Autodesk Inventor part; units mm, degrees
ref_plane "Work Plane1" through (-8.617, 4.975, 0) normal (-0.5, -0.8660254, 0) x (0, 0, -1)
ref_plane "YZ Plane" through (0, 0, 0) normal (1, 0, 0) x (0, 1, 0)
ref_plane "XZ Plane" through (0, 0, 0) normal (0, 1, 0) x (-1, 0, 0)
sketch "Sketch1" plane through (0, 0, 0) normal (0, 0, 1) x (1, 0, 0)
  circle A0 centre (0, 0) radius 30
  circle A1 centre (0, 0) radius 40
  circle A2 centre (0, 0) radius 25
  circle A3 centre (0, 0) radius 13
  circle A4 centre (0, 0) radius 5.5
  circle A5 centre (0, 0) radius 9.95 construction
  line L0 (0, 9.95) -> (8.617, 4.975)
  line L1 (8.617, 4.975) -> (8.617, -4.975)
  line L2 (8.617, -4.975) -> (0, -9.95)
  line L3 (0, -9.95) -> (-8.617, -4.975)
  line L4 (-8.617, -4.975) -> (-8.617, 4.975)
  line L5 (-8.617, 4.975) -> (0, 9.95)
  line L6 (0, 9.95) -> (0, -9.95) construction
  dimension "bolt_head_hub_WAC" = 19.9
  dimension "wheel_diam" = 60
  dimension "d1" = 80
  dimension "d4" = 50
  dimension "d5" = 26
  dimension "hub_id" = 11
extrude "Extrusion1" add sketch "Sketch1" along normal blind 3 contours A0 | A1 | A2 | A3 | A4 | L0 L1 L2 L3 L4 L5
extrude "Extrusion2" add sketch "Sketch1" along normal blind 28 contours A0
extrude "Extrusion3" add sketch "Sketch1" along normal blind 18 contours A3 | L0 L1 L2 L3 L4 L5
extrude "Extrusion4" cut sketch "Sketch1" against normal blind 8.4 from surface at 18 contours L0 L1 L2 L3 L4 L5
extrude "Extrusion5" cut sketch "Sketch1" along normal up to surface (3 mm away) contours A4
fillet "Fillet1" radius 2 1 edges at (-30, 0, 3)
ref_plane "Work Plane1" through (-8.617, 4.975, 0) normal (-0.5, -0.8660254, 0) x (0, 0, -1)
sketch "Sketch3" plane through (-8.617, 4.975, 0) normal (-0.5, -0.8660254, 0) x (0, 0, -1)
  line L0 (-3, 22.95) -> (-18, 22.95)
  line L1 (-3, 34.95) -> (-3, -15.05)
  line L2 (-3, -3.05) -> (-3, 22.95)
  line L3 (-28, 34.95) -> (-3, 34.95)
  line L4 (-18, 22.95) -> (-3, 22.95)
  line L5 (-3, 22.95) -> (-3, 19.95)
  line L6 (-3, 19.95) -> (-18, 19.95)
  line L7 (-18, 19.95) -> (-18, 22.95)
  arc A0 (-18, 22.95) -> (-28, 34.95) centre (-32.838, 20.7516) ccw
  point P0 (0, 9.95)
  dimension "d18" = 3
  dimension "d21" = 15
extrude "Extrusion6" add sketch "Sketch3" along normal mid plane 3
pattern_circular "Circular Pattern1" count 4 over 360 about axis through (0, 0, -10) along (0, 0, 1) of "Extrusion6"
equation "\"bolt_head_hub_WAC\" = bolt_WAC + 2 * printer_tolerance"
equation "\"d1\" = wheel_diam + 2 * flange_extra"
equation "\"d4\" = wheel_diam - 2 * wheel_thick"
equation "\"d5\" = bolt_head_hub_WAC + 2 * bolt_head_hub_clearance"
equation "\"hub_id\" = bolt_od + 2 * printer_tolerance"
equation "\"d8\" = track_w + flange_w"
equation "\"d10\" = flange_w + hub_height"
equation "\"track_w\" = 25"
equation "\"wheel_thick\" = 5"
equation "\"bolt_head_hub_clearance\" = 3.05"
equation "\"hub_height\" = 15"
equation "\"bolt_head_thick\" = 6.4"
equation "\"bolt_WAC\" = 18.9"
equation "\"printer_tolerance\" = 0.5"
properties part number "test_wheel_v1"
CAD build for the part. Positions are in the model's coordinates, mm. Give positions to 0.01 mm unless a question says otherwise; leave off trailing zeros. Order: outer loops, then holes, each group sorted by start corner. A loop starts at its lowest first (then second) coordinate and runs counter-clockwise, first axis right, second up. Notation, with made-up numbers: M -37.75,-6 L -8.75,-6 A17 cw -8.75,22 Z; hole C 10.25,80.5 d3. An arc over 180 degrees is marked long. Put each result on its own line as item: value. Start each with the question number.
(1) Saw through at D-D, the plane z = 19. Write the cut outline in (x, y), then the cut area to 3 significant figures.
(2) Saw through at A-A, the plane z = 7. Write the cut outline in (x, y).
(3) Saw through at B-B, the plane y = 0. Write the cut outline in (x, z).
(4) Saw through at C-C, the plane z = 11.25. Write the cut outline in (x, y) (3 decimals).
(5) Drill centre lines: line 1 along Y through (x, z) = (0, 7.25); line 2 along Y through (x, z) = (-0.5, 21.25) (3 decimals); line 3 along X through (y, z) = (0.5, 10.25) (3 decimals). Where is each one in solid material? Low to high.
(6) Flat gauge pins, fed straight in: pin 1 Ø1 at (x, y) = (-24, 24) entering from +Z; pin 2 Ø10 at (y, z) = (-6.5, 3.5) entering from +X; pin 3 Ø3 at (x, z) = (7.5, 12.5) entering from +Y. Where does each tip first touch, or does it go through?
(7) Mould opens along Y. For faces 1 (the flat face through (-9, 0, 18)), 2 (the cylindrical face through (-8.67, 39.05, 1.48)) say: +Y half, -Y half, draft (parallel to the pull), parting line (faces both ways), or undercut.
Check result:
1. outline: C 0,0 d60; hole M -22.36,11.18 A25 ccw -13.78,-20.86 L -9.59,-13.62 L -7,-15.12 L -11.18,-22.36 A25 ccw 20.86,-13.78 L 13.62,-9.59 L 15.12,-7 L 22.36,-11.18 A25 ccw 13.78,20.86 L 9.59,13.62 L 7,15.12 L 11.18,22.36 A25 ccw -20.86,13.78 L -13.62,9.59 L -15.12,7 Z
1. area: 965 mm2
2. outline: C 0,0 d60; hole M -22.36,11.18 A25 ccw -13.78,-20.86 L -7.76,-10.43 A13 cw -11.93,5.16 Z; hole M -20.86,13.78 L -10.43,7.76 A13 cw 5.16,11.93 L 11.18,22.36 A25 ccw Z; hole M -11.18,-22.36 A25 ccw 20.86,-13.78 L 10.43,-7.76 A13 cw -5.16,-11.93 Z; hole C 0,0 d11; hole M 7.76,10.43 A13 cw 11.93,-5.16 L 22.36,-11.18 A25 ccw 13.78,20.86 Z
3. outline: M -40,0 L -5.5,0 L -5.5,9.6 L -8.62,9.6 L -8.62,18 L -13,18 L -13,3 L -25,3 L -25,28 L -30,28 L -30,5 A2 cw -32,3 L -40,3 Z; M 5.5,0 L 40,0 L 40,3 L 32,3 A2 cw 30,5 L 30,28 L 25,28 L 25,3 L 13,3 L 13,18 L 8.62,18 L 8.62,9.6 L 5.5,9.6 Z
4. outline: C 0,0 d60; hole M -22.362,11.178 A25 ccw -13.777,-20.862 L -7.756,-10.433 A13 cw -11.933,5.158 Z; hole M -20.862,13.777 L -10.433,7.756 A13 cw 5.158,11.933 L 11.178,22.362 A25 ccw Z; hole M -11.178,-22.362 A25 ccw 20.862,-13.777 L 10.433,-7.756 A13 cw -5.158,-11.933 Z; hole M -8.617,-4.975 L 0,-9.95 L 8.617,-4.975 L 8.617,4.975 L 0,9.95 L -8.617,4.975 Z; hole M 7.756,10.433 A13 cw 11.933,-5.158 L 22.362,-11.178 A25 ccw 13.777,20.862 Z
5. line 1: y = -30 to -25, -13 to -5.5, 5.5 to 13, 25 to 30
5. line 2: y = -29.996 to -24.995, 24.995 to 29.996
5. line 3: x = -29.996 to -24.995, -12.99 to -8.617, 8.617 to 12.99, 24.995 to 29.996
6. pin 1: stops at z = 3
6. pin 2: stops at x = 39.97
6. pin 3: stops at y = 29.39
7. face 1: undercut
7. face 2: parting line
